```python
from build123d import *

# Parameters (mm, degrees)
F0_W     = 100
F0_H     = 100
F2_DEPTH = 10
F4_SIZE2 = 5
F4_SIZE  = 5
F3_W     = 10
F3_H     = 10
F5_DEPTH = 34
F6_DEPTH = 2
F7_SIZE  = 1
F8_W     = 5
F8_H     = 4.9
F8_H_2   = 5
F9_DEPTH = 100


with BuildPart() as f2:
    # F0 (on Top) → F2 (new body)
    with BuildSketch(Plane.XY):
        with Locations((0.868328, 4.095532)):
            Rectangle(F0_W, F0_H)
    extrude(amount=-F2_DEPTH)

    # F4
    f4_edges = [f2.edges().sort_by_distance(p)[0] for p in [
        (0.868328, -45.904468, 0),
        (-49.131672, 4.095532, 0),
        (0.868328, 54.095532, 0),
        (50.868328, 4.095532, 0),
    ]]
    chamfer(f4_edges, length=F4_SIZE, length2=F4_SIZE2)

    # F3 (on face) → F5 (cut)
    with BuildSketch(Plane.XY):
        with Locations((35.868328, 39.095532)):
            Rectangle(F3_W, F3_H)
    extrude(amount=-F5_DEPTH, mode=Mode.SUBTRACT)

    # F1 (on face) → F6 (cut)
    with BuildSketch(Plane.XY):
        Polygon((-7.571068, 17.362981), (-17.631035, 6.923928), (-17.362981, -7.571068), (-6.923928, -17.631035), (7.571068, -17.362981), (17.631035, -6.923928), (17.362981, 7.571068), (6.923928, 17.631035), align=None)
    extrude(amount=-F6_DEPTH, mode=Mode.SUBTRACT)

    # F7
    f7_edges = [f2.edges().sort_by_distance(p)[0] for p in [
        (12.143455, 12.601052, -2),
        (-0.32357, 17.497008, -2),
        (-12.601052, 12.143455, -2),
        (-17.497008, -0.32357, -2),
        (-12.143455, -12.601052, -2),
        (0.32357, -17.497008, -2),
        (12.601052, -12.143455, -2),
        (17.497008, 0.32357, -2),
    ]]
    chamfer(f7_edges, length=F7_SIZE)

    # F8 (on face) → F9 (join)
    with BuildSketch(Plane(origin=(0, 0, -10), x_dir=(1, 0, 0), z_dir=(0, 0, -1))):
        with Locations((-46.631672, -51.645532)):
            Rectangle(F8_W, F8_H)
        with Locations((-46.631672, 43.404468)):
            Rectangle(F8_W, F8_H_2)
        with Locations((47.968328, -51.645532)):
            Rectangle(F8_W, F8_H)
        with Locations((47.968328, 43.404468)):
            Rectangle(F8_W, F8_H_2)
    extrude(amount=F9_DEPTH)


solid = f2.part
```
Input: part model. Units: mm. Frame: model coordinates. A direction names the side the tool comes from. Give positions to 0.01 mm unless a question says otherwise; leave off trailing zeros. Order: outer loops, then holes, each group sorted by start corner. A loop starts at its lowest first (then second) coordinate and runs counter-clockwise, first axis right, second up.
1. Cut plane D-D (x = -22). Return loops of the section in (y, z).
Computed:
outline: (-45.9, -10) - (54.1, -10) - (54.1, -5) - (49.1, 0) - (-40.9, 0) - (-45.9, -5) - close
2. Draft query along X for faces 6 (the face through (-46.6, 3.4, -2.47)), 7 (the face through (-44.132, 52, -59)), 8 (the face through (-47, 52, -110)), 9 (the face through (0, 0, -2)). Return one class per face: released by +X, released by -X, zero draft, split by the parting line, or undercut.
Computed:
face 6: released by -X
face 7: undercut
face 8: zero draft
face 9: undercut
3. Cut plane C-C (y = 41.5). Return loops of the section in (x, z), and give its area (3 significant figures).
Computed:
outline: (-49.13, -10) - (30.87, -10) - (30.87, 0) - (-44.13, 0) - (-49.13, -5) - close; (40.87, -10) - (50.87, -10) - (50.87, -5) - (45.87, 0) - (40.87, 0) - close
area: 875 mm2
4. Cut plane A-A (x = 38). Return loops of the section in (y, z), and give its area (3 significant figures).
Computed:
outline: (-45.9, -10) - (34.1, -10) - (34.1, 0) - (-40.9, 0) - (-45.9, -5) - close; (44.1, -10) - (54.1, -10) - (54.1, -5) - (49.1, 0) - (44.1, 0) - close
area: 875 mm2
5. Line query: probe 1 along Y at (x, z) = (47.5, -82.5); probe 2 along Z at (x, y) = (-24, 14); probe 3 along Y at (x, z) = (35.5, -7.5). Output: solid intervals per line, ascending.
Computed:
probe 1: y = -45.9 to -40.9, 49.2 to 54.1
probe 2: z = -10 to 0
probe 3: y = -45.9 to 34.1, 44.1 to 54.1
6. Set-up query: faces 1 (the face through (50.468, -43, -59)), 2 (the face through (48, -40.904, -59)), 3 (the face through (40.868, 39, -5)), 4 (the face through (-11.865, -12.166, -1.507)), 5 (the face through (45.468, -43, -59)). Return all of +Z, -Z, +X, -X, +Y, -Y with unobstructed straight access to the full face (end or side cutting, diameter ignored); none if empty.
Computed:
face 1: -Z, +X, +Y, -Y
face 2: -Z, +X, -X
face 3: +Z, -Z
face 4: +Z
face 5: -Z, +Y, -Y
7. Pin query (flat end, axial travel): pin 1 Ø8 at (x, y) = (1.5, 27) entering from -Z; pin 2 Ø5.5 at (y, z) = (50.5, -36.5) entering from +X. Return the tip coordinate at first contact, or that it passes through.
Computed:
pin 1: stops at z = -10
pin 2: stops at x = 50.47
8. Cut plane B-B (z = -34). Return loops of the section in (x, y), and give its area (3 significant figures).
Computed:
outline: (-49.13, -45.9) - (-44.13, -45.9) - (-44.13, -40.9) - (-49.13, -40.9) - close; (-49.13, 49.2) - (-44.13, 49.2) - (-44.13, 54.1) - (-49.13, 54.1) - close; (45.47, -45.9) - (50.47, -45.9) - (50.47, -40.9) - (45.47, -40.9) - close; (45.47, 49.2) - (50.47, 49.2) - (50.47, 54.1) - (45.47, 54.1) - close
area: 99.0 mm2
